```python
from build123d import *

# Parameters (mm, degrees)
F0_W      = 88
F0_H      = 18
F1_DEPTH  = 23
F2_W      = 74
F2_H      = 18
F3_DEPTH  = 20
F5_DEPTH  = 4
F7_DEPTH  = 4
F8_R      = 2.5
F9_DEPTH  = 3
F10_R     = 2.5
F11_DEPTH = 3
F12_W     = 88
F12_H     = 18
F13_DEPTH = 3
F15_R     = 5


with BuildPart() as f1:
    # F0 (on Top) → F1 (new body)
    with BuildSketch(Plane.XY):
        Rectangle(F0_W, F0_H)
    extrude(amount=F1_DEPTH)

    # F2 (on face) → F3 (cut)
    with BuildSketch(Plane.XY.offset(23)):
        Rectangle(F2_W, F2_H)
    extrude(amount=-F3_DEPTH, mode=Mode.SUBTRACT)

    # F4 (on face) → F5 (cut)
    with BuildSketch(Plane(origin=(37, 0, 0), x_dir=(0, -1, 0), z_dir=(-1, 0, 0))):
        Polygon((-2.309401, 9), (2.309401, 9), (4.618802, 13), (2.309401, 17), (-2.309401, 17), (-4.618802, 13), align=None)
    extrude(amount=-F5_DEPTH, mode=Mode.SUBTRACT)

    # F6 (on face) → F7 (cut)
    with BuildSketch(Plane.YZ.offset(-37)):
        Polygon((-2.309401, 9), (2.309401, 9), (4.618802, 13), (2.309401, 17), (-2.309401, 17), (-4.618802, 13), align=None)
    extrude(amount=-F7_DEPTH, mode=Mode.SUBTRACT)

    # F8 (on face) → F9 (cut, through all)
    with BuildSketch(Plane(origin=(41, 0, 0), x_dir=(0, -1, 0), z_dir=(-1, 0, 0))):
        with Locations((0, 13)):
            Circle(F8_R)
    extrude(amount=-F9_DEPTH, mode=Mode.SUBTRACT)

    # F10 (on face) → F11 (cut, through all)
    with BuildSketch(Plane.YZ.offset(-41)):
        with Locations((0, 13)):
            Circle(F10_R)
    extrude(amount=-F11_DEPTH, mode=Mode.SUBTRACT)


with BuildPart() as f13:
    # F12 (on face) → F13 (new body)
    with BuildSketch(Plane.XY.offset(23)):
        Rectangle(F12_W, F12_H)
    extrude(amount=F13_DEPTH)


with BuildPart() as f1_1:
    add(f1.part)

    # F14: union F13
    add(f13.part)

    # F15
    f15_edges = [f1_1.edges().sort_by_distance(p)[0] for p in [
        (-44, 0, 26),
        (-44, 0, 0),
        (44, 0, 26),
        (44, 0, 0),
        (-44, -9, 13),
        (-44, 9, 13),
        (44, -9, 13),
        (44, 9, 13),
    ]]
    fillet(f15_edges, radius=F15_R)


solid = f1_1.part
```
Could you check a few things on this model? Use its own coordinates, in mm. A direction names the side the tool comes from. Coordinates: 2 decimals unless noted, no trailing zeros. Order: outer loops, then holes, each group sorted by start corner. A loop starts at its lowest first (then second) coordinate and runs counter-clockwise, first axis right, second up. Notation, with made-up numbers: M 6,77 L 46,77 A20 ccw 46,95 Z; hole C 3.5,-14.5 d4. An arc over 180 degrees is marked long. Use one line per item in the form item = value. Start each with the question number.
1. For pin 1 (12 mm diameter, centred on x = -17, z = 3.5, fed in from +Y); pin 2 (3 mm diameter, centred on y = 0, z = 13, fed in from -X); pin 3 (1.2 mm diameter, centred on x = -40, y = 0.5, fed in from +Z); pin 4 (1 mm diameter, centred on y = 7, z = 10, fed in from -X), each with a flat end and sliding along its axis, tell me the tip position at first contact or that it passes through.
2. On a 3-axis mill with a long thin cutter (end or side, diameter ignored), from which of +Z, -Z, +X, -X, +Y, -Y can I reach the whole of each face in a straight line? I mean faces 4 (the flat face through (38.972, 3.448, 15.028)), 5 (the flat face through (-1, 0, 23)), 6 (the flat face through (-3, -9, 24)). Say none if no direction works.
3. Suppose I cut it at A-A on z = 5.75. Write out the boundary of the cut face in (x, y).
4. Suppose I cut it at D-D on x = 38. Write out the boundary of the cut face in (y, z).
5. Suppose I cut it at C-C on y = 0. Write out the boundary of the cut face in (x, z).
6. We'd pull the mould along Y, two halves only. Please class faces 1 (the flat face through (44, -2, 11)), 2 (the flat face through (41, -2, 15)), 3 (the cylindrical face through (43, -7, 13)): +Y half, -Y half, draft (parallel to the pull), parting line (faces both ways), or undercut.
7. Suppose I cut it at B-B on x = 20. Write out the boundary of the cut face in (y, z).
8. Please list where these lines run through material, in increasing order: line 1 (Z direction, x = 11, y = -3); line 2 (X direction, y = 7, z = 22.25); line 3 (X direction, y = -3, z = 4.5).
Geometry says:
q1.pin_1 = 9
q1.pin_2 = through
q1.pin_3 = 25.98
q1.pin_4 = -43.33
q2.face_4 = none
q2.face_5 = +Y, -Y
q2.face_6 = +Z, -Z, +X, -X, -Y
q3.outline = M -44,-4 A5 ccw -39,-9 L -37,-9 L -37,9 L -39,9 A5 ccw -44,4 Z; M 37,-9 L 39,-9 A5 ccw 44,-4 L 44,4 A5 ccw 39,9 L 37,9 Z
q4.outline = M -9,0 L 9,0 L 9,26 L -9,26 Z; hole M -4.62,13 L -2.31,9 L 2.31,9 L 4.62,13 L 2.31,17 L -2.31,17 Z
q5.outline = M -44,5 A5 ccw -39,0 L 39,0 A5 ccw 44,5 L 44,10.5 L 41,10.5 L 41,9 L 37,9 L 37,3 L -37,3 L -37,9 L -41,9 L -41,10.5 L -44,10.5 Z; M -44,15.5 L -41,15.5 L -41,17 L -37,17 L -37,23 L 37,23 L 37,17 L 41,17 L 41,15.5 L 44,15.5 L 44,21 A5 ccw 39,26 L -39,26 A5 ccw -44,21 Z
q6.face_1 = draft
q6.face_2 = undercut
q6.face_3 = -Y half
q7.outline = M -9,0 L 9,0 L 9,3 L -9,3 Z; M -9,23 L 9,23 L 9,26 L -9,26 Z
q8.line_1 = 0 to 3, 23 to 26
q8.line_2 = -43 to -37, 37 to 43
q8.line_3 = -43.97 to -37, 37 to 43.97
